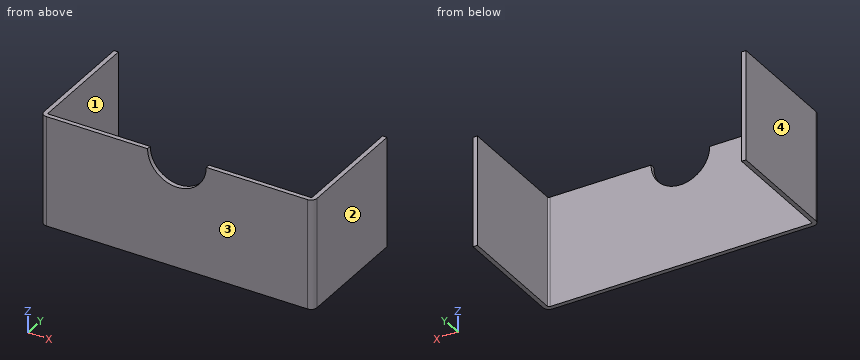
from build123d import *

# Parameters (mm, degrees)
BRIDA_BASE1_DEPTH     = 75
CROQUIS6_R            = 20
CORTAR_EXTRUIR1_DEPTH = 10


# Sheet-metal steps are written as plain solids
with BuildPart() as part:
    # Croquis1 → Brida base1 (new body)
    with BuildSketch(Plane.XY):
        with BuildLine():
            Line((180, 80), (180, 1))
            ThreePointArc((180, 1), (179.707106781, 0.292893219), (179, 0))
            Line((179, 0), (1, 0))
            ThreePointArc((1, 0), (0.292893219, 0.292893219), (0, 1))
            Line((0, 1), (0, 80))
            Line((0, 80), (-3, 80))
            Line((-3, 80), (-3, 1))
            ThreePointArc((-3, 1), (-1.828427125, -1.828427125), (1, -3))
            Line((1, -3), (179, -3))
            ThreePointArc((179, -3), (181.828427125, -1.828427125), (183, 1))
            Line((183, 1), (183, 80))
            Line((183, 80), (180, 80))
        make_face()
    extrude(amount=BRIDA_BASE1_DEPTH)

    # Croquis6 → Cortar-Extruir1 (cut)
    with BuildSketch(Plane(origin=(0, 0, 0), x_dir=(1, 0, 0), z_dir=(0, 1, 0))):
        with Locations((90, -75)):
            Circle(CROQUIS6_R)
    extrude(amount=-CORTAR_EXTRUIR1_DEPTH, mode=Mode.SUBTRACT)


solid = part.part
Model file for the job. Use its own axes, mm. Face numbers are marked on the shaded views. Give positions to 0.01 mm unless a question says otherwise; leave off trailing zeros. Loops run counter-clockwise (first coordinate to the right, second up) from the corner with the lowest first, then second, coordinate; pieces in that order, holes last.
1) Saw through at C-C (z = 14). Write the cut outline in (x, y), plus the area to 3 significant figures.
2) Saw through at A-A (z = 59). Write the cut outline in (x, y), plus the area to 3 significant figures.
3) Flat gauge pin, fed straight in: pin 1 Ø2 at (x, z) = (20, 40.5) entering from +Y. Where does the tip first touch, or does it go through?
4) Saw through at B-B (y = 13.5). Write the cut outline in (x, z).
5) Wall check: line 1 (X direction, y = 72, z = 31.5); line 2 (Y direction, x = 16, z = 6.5). Give the ranges that are in metal, low to high.
6) Saw through at D-D (x = 90). Write the cut outline in (y, z), plus the area to 3 significant figures.
7) Pull direction X, two halves, no side cores. Call the marked faces 1, 2, 3 and 4: +X half, -X half, draft (parallel to the pull), parting line (faces both ways), or undercut.
Answer block:
1. outline: (-3, 1) arc R4 ccw to (1, -3) - (179, -3) arc R4 ccw to (183, 1) - (183, 80) - (180, 80) - (180, 1) arc R1 cw to (179, 0) - (1, 0) arc R1 cw to (0, 1) - (0, 80) - (-3, 80) - close
1. area: 1,030 mm2
2. outline: (-3, 1) arc R4 ccw to (1, -3) - (78, -3) - (78, 0) - (1, 0) arc R1 cw to (0, 1) - (0, 80) - (-3, 80) - close; (102, -3) - (179, -3) arc R4 ccw to (183, 1) - (183, 80) - (180, 80) - (180, 1) arc R1 cw to (179, 0) - (102, 0) - close
2. area: 960 mm2
3. pin 1: stops at y = 0
4. outline: (-3, 0) - (0, 0) - (0, 75) - (-3, 75) - close; (180, 0) - (183, 0) - (183, 75) - (180, 75) - close
5. line 1: x = -3 to 0, 180 to 183
5. line 2: y = -3 to 0
6. outline: (-3, 0) - (0, 0) - (0, 55) - (-3, 55) - close
6. area: 165 mm2
7. face 1: undercut
7. face 2: +X half
7. face 3: draft
7. face 4: -X half
